from build123d import *

# Parameters (mm, degrees)
PAD001_DEPTH            = 27.625
SKETCH006_W             = 4
SKETCH006_H             = 40.3
POCKET003_DEPTH         = 19
SKETCH007_W             = 11
SKETCH007_H             = 7.48
POCKET004_DEPTH         = 161.659754
SKETCH008_R             = 2
POCKET005_DEPTH         = 5
POCKET006_DEPTH         = 2.3
SKETCH010_R             = 2
POCKET007_DEPTH         = 1.7
FILLET001_R             = 3
FILLET002_R             = 2.5
BODY001_PLACEMENT_ANGLE = 90
SKETCH_R                = 40
PAD_DEPTH               = 15
POCKET_DEPTH            = 3.5
SKETCH002_R             = 3.25
POCKET001_DEPTH         = 8.5
SKETCH003_R             = 1.75
POCKET002_DEPTH         = 15.001
FILLET_R                = 3
FILLET003_R             = 1


with BuildPart() as body001:
    # Sketch005 → Pad001 (new body, symmetric)
    with BuildSketch(Plane.YZ):
        Polygon((-17.5, 23), (-17.5, 0), (17.5, 0), (17.5, 23), (13.5, 23), (13.5, 4), (-13.5, 4), (-13.5, 23), align=None)
    extrude(amount=PAD001_DEPTH, both=True)

    # Sketch006 (on Face8 of Pad001) → Pocket003 (cut)
    with BuildSketch(Plane(origin=(0, 0, 23), x_dir=(0, -1, 0), z_dir=(0, 0, 1))):
        with Locations((15.5, 0)):
            Rectangle(SKETCH006_W, SKETCH006_H)
    extrude(amount=-POCKET003_DEPTH, mode=Mode.SUBTRACT)

    # Sketch007 (on Face11 of Pocket003) → Pocket004 (cut, through all)
    with BuildSketch(Plane(origin=(0, 0, 23), x_dir=(0, -1, 0), z_dir=(0, 0, 1))):
        with Locations((-12, 23.885)):
            Rectangle(SKETCH007_W, SKETCH007_H)
    pocket004 = extrude(amount=-POCKET004_DEPTH, mode=Mode.SUBTRACT)

    # Mirrored: Pocket004 across YZ
    add(pocket004.mirror(Plane.YZ), mode=Mode.SUBTRACT)

    # Sketch008 (on Face1 of Mirrored) → Pocket005 (cut)
    with BuildSketch(Plane(origin=(0, -17.5, 0), x_dir=(0, 0, -1), z_dir=(0, -1, 0))):
        with Locations((-19.01, -24.475)):
            Circle(SKETCH008_R)
        with Locations((-8.99, -24.475)):
            Circle(SKETCH008_R)
        with Locations((-8.99, 24.475)):
            Circle(SKETCH008_R)
        with Locations((-19.01, 24.475)):
            Circle(SKETCH008_R)
    extrude(amount=-POCKET005_DEPTH, mode=Mode.SUBTRACT)

    # Sketch009 (on Face22 of Pocket005) → Pocket006 (cut)
    with BuildSketch(Plane(origin=(0, 13.5, 0), x_dir=(0, 0, -1), z_dir=(0, -1, 0))):
        Polygon((-11.598815, -11.77), (-11.598815, -8.42), (-14.5, -6.745), (-17.401185, -8.42), (-17.401185, -11.77), (-14.5, -13.445), align=None)
    extrude(amount=-POCKET006_DEPTH, mode=Mode.SUBTRACT)

    # Sketch010 (on Face30 of Pocket006) → Pocket007 (cut)
    with BuildSketch(Plane(origin=(0, 15.8, 0), x_dir=(0, 0, -1), z_dir=(0, -1, 0))):
        with Locations((-14.5, -10.095)):
            Circle(SKETCH010_R)
    extrude(amount=-POCKET007_DEPTH, mode=Mode.SUBTRACT)

    # Fillet001
    fillet001_edges = [body001.edges().sort_by_distance(p)[0] for p in [
        (-20.15, -15.5, 23),
        (-27.625, -15.5, 23),
        (20.15, -15.5, 23),
        (27.625, -15.5, 23),
        (20.145, 15.5, 23),
        (27.625, 6.5, 2),
        (-20.145, 15.5, 23),
        (-27.625, 6.5, 2),
        (-20.145, 6.5, 2),
        (20.145, 6.5, 2),
        (0, 13.5, 4),
    ]]
    fillet(fillet001_edges, radius=FILLET001_R)

    # Fillet002
    fillet002_edges = [body001.edges().sort_by_distance(p)[0] for p in [
        (-23.8875, -13.5, 4),
        (23.8875, -13.5, 4),
    ]]
    fillet(fillet002_edges, radius=FILLET002_R)


with BuildPart() as body001_1:
    # Body001 placement: moved
    add(body001.part.moved(Location((0, 0, 15))).rotate(Axis((0, 0, 15), (0, 0, 1)), BODY001_PLACEMENT_ANGLE))


with BuildPart() as body:
    # Sketch → Pad (new body)
    with BuildSketch(Plane.XY):
        Circle(SKETCH_R)
    extrude(amount=PAD_DEPTH)

    # Sketch001 (on Face2 of Pad) → Pocket (cut)
    with BuildSketch(Plane(origin=(0, 0, 0), x_dir=(1, 0, 0), z_dir=(0, 0, -1))):
        Polygon((2.875, -4.979646), (5.75, 0), (2.875, 4.979646), (-2.875, 4.979646), (-5.75, 0), (-2.875, -4.979646), align=None)
    extrude(amount=-POCKET_DEPTH, mode=Mode.SUBTRACT)

    # Sketch002 (on Face10 of Pocket) → Pocket001 (cut)
    with BuildSketch(Plane(origin=(0, 0, 3.5), x_dir=(1, 0, 0), z_dir=(0, 0, -1))):
        Circle(SKETCH002_R)
    extrude(amount=-POCKET001_DEPTH, mode=Mode.SUBTRACT)

    # Sketch003 (on Face3 of Pocket001) → Pocket002 (cut, through all)
    with BuildSketch(Plane.XY.offset(15)):
        with Locations((22.3, 0)):
            Circle(SKETCH003_R)
        with Locations((-22.3, 0)):
            Circle(SKETCH003_R)
    extrude(amount=-POCKET002_DEPTH, mode=Mode.SUBTRACT)

    # Fillet
    fillet_edges = [body.edges().sort_by_distance(p)[0] for p in [
        (-40, 0, 15),
    ]]
    fillet(fillet_edges, radius=FILLET_R)

    # Boolean: union Body001
    add(body001_1.part)

    # Fillet003
    fillet003_edges = [body.edges().sort_by_distance(p)[0] for p in [
        (17.5, 0, 15),
        (7, 27.625, 15),
        (7, -27.625, 15),
        (-17.5, 0, 15),
    ]]
    fillet(fillet003_edges, radius=FILLET003_R)


solid = body.part
For this review, take the finished solid that the model builds, in its own axes (mm). A direction names the side the tool comes from. Round coordinates to 2 decimals unless told otherwise and drop trailing zeros. Loops run counter-clockwise (first coordinate to the right, second up) from the corner with the lowest first, then second, coordinate; pieces in that order, holes last. Notation, with made-up numbers: (61, 18.25) - (79, 18.25) arc R24 cw to (79, 43.25) - close; hole circle Ø3 at (20.25, 16.5). An arc over 180 degrees is marked (long way). One line per item, written item: value. Start each with the question number.
Item 1: For faces 4 (the flat face through (4.292, 2.525, 1.726)), 5 (the flat face through (3, 0, 19)), 6 (the flat face through (13.5, -24, 30)), 7 (the flat face through (-14.634, -7.594, 28.029)), 8 (the flat face through (-15, 20.145, 26)), list the 3-axis set-ups (+Z, -Z, +X, -X, +Y, -Y) from which the entire face can be reached by the end or side of a thin tool; tool diameter is ignored.
Item 2: For L1, parallel to Y at x = 16, z = 34 (3 decimals); L2, parallel to Z at x = -6.5, y = -6.5; L3, parallel to Z at x = 24.5, y = 23, list the stretches that pass through material, from the lowest coordinate up.
Item 3: Take a section at A-A (z = 23.99). Give the boundary of the cut face in (x, y) (3 decimals).
Item 4: Take a section at B-B (z = 6). Give the boundary of the cut face in (x, y).
Item 5: The part is to be moulded in two halves that separate along Y. For faces 1 (the flat face through (17.5, -2, 18)), 2 (the flat face through (-15, -20.145, 26)), 3 (the flat face through (-15.8, -12.3, 29.5)), say which applies: +Y half, -Y half, draft (parallel to the pull), parting line (faces both ways), or undercut.
Item 6: Clearance check with flat-ended pins moving along their axes: pin 1 Ø6 at (y, z) = (22.5, 29.5) entering from -X; pin 2 Ø5 at (y, z) = (2, 26.5) entering from +X; pin 3 Ø3 at (x, y) = (-21, 11.5) entering from +Z. State where each tip first meets the part, or that it passes through.
Answer below:
1. face 4: -Z
1. face 5: +Z
1. face 6: +Z, -X, +Y, -Y
1. face 7: +X
1. face 8: +Z, -X, +Y
2. L1: y = -27.625 to -26.475, -22.475 to -20.15, 20.15 to 22.475, 26.475 to 27.625
2. L2: z = 0 to 19
2. L3: z = 0 to 15
3. outline: (-17.5, -20.145) - (-13.5, -20.145) - (-13.5, 20.145) - (-17.5, 20.145) - close; (13.5, -27.625) - (17.5, -27.625) - (17.5, -26.475) - (13.5, -26.475) - close; (13.5, -22.475) - (17.5, -22.475) - (17.5, -20.15) - (13.5, -20.15) - close; (13.5, 20.15) - (17.5, 20.15) - (17.5, 22.475) - (13.5, 22.475) - close; (13.5, 26.475) - (17.5, 26.475) - (17.5, 27.625) - (13.5, 27.625) - close
4. outline: circle Ø80 at (0, 0); hole circle Ø3.5 at (-22.3, 0); hole circle Ø6.5 at (0, 0); hole circle Ø3.5 at (22.3, 0)
5. face 1: draft
5. face 2: -Y half
5. face 3: undercut
6. pin 1: stops at x = -17.5
6. pin 2: stops at x = -13.5
6. pin 3: stops at z = 15
